The figure shows three views and two pictorial views of one solid part (mm, origin at its lowest corner). Answer the questions. Round coordinates to 2 decimals unless told otherwise and drop trailing zeros. Order: outer loops, then holes, each group sorted by start corner. A loop starts at its lowest first (then second) coordinate and runs counter-clockwise, first axis right, second up. Notation, with made-up numbers: (59.25, 84.5) -> (97.25, 84.5) arc R18 cw to (97.25, 92.5) -> close; hole circle Ø9 at (61, 86). An arc over 180 degrees is marked (long way). Answer as a JSON object with one key per item and string values. Group by question number.
Item 1: Given P1, Ø1, axis at y = 1.5, z = 4, coming from the +X side; P2, Ø1.6, axis at y = 2.5, z = 3.5, coming from the -X side, each flat-ended and moving along its own axis, determine where each tip first touches the part or whether it passes through.
Item 2: Section C-C, the plane z = 3.5 is taken. Write down the section's boundary in (x, y) (1 decimal), plus the area to 3 significant figures.
Item 3: Section A-A, the plane y = 1.4 is taken. Write down the section's boundary in (x, z) (1 decimal), plus the area to 3 significant figures.
Item 4: Section B-B, the plane x = 53 is taken. Write down the section's boundary in (y, z) (1 decimal).
Item 5: Consider probe 1 along X at (y, z) = (1.5, 4.75); probe 2 along Z at (x, y) = (35, 3.05) (1 decimal); probe 3 along X at (y, z) = (2.7, 3.25). Determine where each line is inside the solid, lowest interval first. Write a range as from..to.
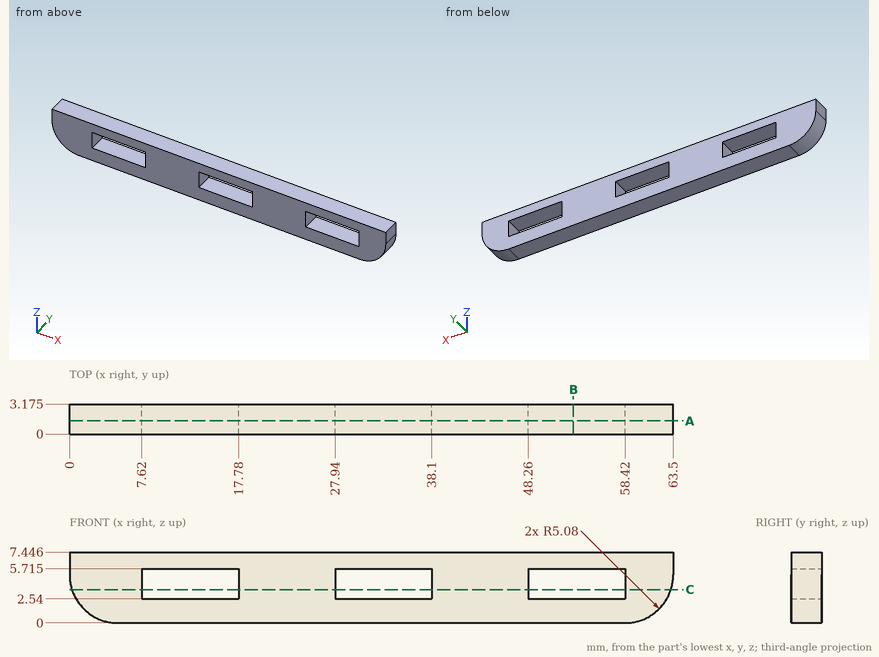
Values found:
{
 "1": {"P1": "x = 63.47", "P2": "x = 0.06"},
 "2": {"outline": "(0.3, 0) -> (7.6, 0) -> (7.6, 3.2) -> (0.3, 3.2) -> close; (17.8, 0) -> (27.9, 0) -> (27.9, 3.2) -> (17.8, 3.2) -> close; (38.1, 0) -> (48.3, 0) -> (48.3, 3.2) -> (38.1, 3.2) -> close; (58.4, 0) -> (63.2, 0) -> (63.2, 3.2) -> (58.4, 3.2) -> close", "area": "103 mm2"},
 "3": {"outline": "(0, 5.1) arc R5.1 ccw to (5.1, 0) -> (58.4, 0) arc R5.1 ccw to (63.5, 5.1) -> (63.5, 7.4) -> (0, 7.4) -> close; hole (7.6, 2.5) -> (17.8, 2.5) -> (17.8, 5.7) -> (7.6, 5.7) -> close; hole (27.9, 2.5) -> (38.1, 2.5) -> (38.1, 5.7) -> (27.9, 5.7) -> close; hole (48.3, 2.5) -> (58.4, 2.5) -> (58.4, 5.7) -> (48.3, 5.7) -> close", "area": "365 mm2"},
 "4": {"outline": "(0, 0) -> (3.2, 0) -> (3.2, 2.5) -> (0, 2.5) -> close; (0, 5.7) -> (3.2, 5.7) -> (3.2, 7.4) -> (0, 7.4) -> close"},
 "5": {"probe 1": "0.01..7.62, 17.78..27.94, 38.1..48.26, 58.42..63.49", "probe 2": "0..2.5, 5.7..7.4", "probe 3": "0.34..7.62, 17.78..27.94, 38.1..48.26, 58.42..63.16"}
}
